CAD build for the part. Positions are in the model's coordinates, mm. A direction names the side the tool comes from. Round coordinates to 2 decimals unless told otherwise and drop trailing zeros. Loops run counter-clockwise (first coordinate to the right, second up) from the corner with the lowest first, then second, coordinate; pieces in that order, holes last.
```python
from build123d import *

# Parameters (mm, degrees)
SKETCH1_R             = 8.5
SKETCH1_R_2           = 6.5
BOSS_EXTRUDE1_DEPTH   = 9
SKETCH1_R_3           = 2.25
SKETCH1_R_4           = 0.75
BOSS_EXTRUDE1_2_DEPTH = 9
SKETCH2_R             = 9.5
BOSS_EXTRUDE2_DEPTH   = 1.5
SKETCH3_R             = 9.5
SKETCH3_R_2           = 6.5
BOSS_EXTRUDE3_DEPTH   = 1
BOSS_EXTRUDE4_REACH   = 19.051
CIRPATTERN1_COUNT     = 3
CUT_EXTRUDE2_START    = -2
SKETCH6_R             = 6.5
CUT_EXTRUDE2_DEPTH    = 2
FILLET1_R             = 3
BOSS_EXTRUDE5_START   = 1
SKETCH8_R             = 6.5
BOSS_EXTRUDE5_DEPTH   = 1
SKETCH11_R            = 8
BOSS_EXTRUDE6_DEPTH   = 2
SKETCH7_R             = 1
CUT_EXTRUDE3_DEPTH    = 7
FILLET2_R             = 1
CIRPATTERN2_COUNT     = 3
CUT_EXTRUDE4_START    = -20
SKETCH4_R             = 0.75
CUT_EXTRUDE4_DEPTH    = 20


with BuildPart() as part:
    # Sketch1 → Boss-Extrude1 (new body)
    with BuildSketch(Plane.XY):
        Circle(SKETCH1_R)
        Circle(SKETCH1_R_2, mode=Mode.SUBTRACT)
    extrude(amount=BOSS_EXTRUDE1_DEPTH)



with BuildPart() as body_2:
    # Sketch1 → Boss-Extrude1 2 (new body)
    with BuildSketch(Plane.XY):
        Circle(SKETCH1_R_3)
        Circle(SKETCH1_R_4, mode=Mode.SUBTRACT)
    extrude(amount=BOSS_EXTRUDE1_2_DEPTH)


with BuildPart() as part_1:
    add(part.part)

    add(body_2.part)  # Boss-Extrude2 merges body 2
    # Sketch2 → Boss-Extrude2 (add)
    with BuildSketch(Plane(origin=(0, 0, 0), x_dir=(-1, 0, 0), z_dir=(0, 0, -1))):
        Circle(SKETCH2_R)
    extrude(amount=BOSS_EXTRUDE2_DEPTH)

    # Sketch3 → Boss-Extrude3 (add)
    with BuildSketch(Plane.XY.offset(9)):
        Circle(SKETCH3_R)
        Circle(SKETCH3_R_2, mode=Mode.SUBTRACT)
    extrude(amount=BOSS_EXTRUDE3_DEPTH)

    # Sketch5 → Boss-Extrude4 (add, up to next)
    with BuildSketch(Plane.XY.offset(9), mode=Mode.PRIVATE) as boss_extrude4_sk1:
        with BuildLine():
            Line((2.25, 0), (6.5, 0))
            ThreePointArc((6.5, 0), (6.444391599, -0.848420249), (6.278517871, -1.682323793))
            Line((6.278517871, -1.682323793), (2.173333109, -0.582342851))
            ThreePointArc((2.173333109, -0.582342851), (2.230750938, -0.293683932), (2.25, 0))
        make_face()
    boss_extrude4_tool1 = extrude(boss_extrude4_sk1.sketch, amount=-BOSS_EXTRUDE4_REACH, mode=Mode.PRIVATE) - part_1.part
    boss_extrude4 = boss_extrude4_tool1.solids().sort_by_distance((4.665326, -0.614202, 9))[0]
    add(boss_extrude4)

    # CirPattern1: Boss-Extrude4 ×3 about axis
    cirpattern1_axis = Axis((0, 0, 0), (0, 0, 1))
    for i in range(1, CIRPATTERN1_COUNT):
        add(boss_extrude4.rotate(cirpattern1_axis, i * 360 / CIRPATTERN1_COUNT))

    # Sketch6 → Cut-Extrude2 (cut)
    with BuildSketch(Plane.XY.offset(9).offset(CUT_EXTRUDE2_START)):
        Circle(SKETCH6_R)
    extrude(amount=CUT_EXTRUDE2_DEPTH, mode=Mode.SUBTRACT)

    # Fillet1
    # the kernel refuses this fillet: 3 mm, written as the material it adds along each edge
    with BuildSketch(Plane(origin=(0, 0, 7), x_dir=(0.9659258262890711, -0.2588190451025104, 0), z_dir=(-0.2588190451025104, -0.9659258262890711, 0))) as fillet1_piece_1:
        with BuildLine():
            CenterArc((6.5 - FILLET1_R, FILLET1_R), FILLET1_R, 270, 90)
            Line((6.5 - FILLET1_R, 0), (6.5, 0))
            Line((6.5, 0), (6.5, FILLET1_R))
        make_face()
    revolve(axis=Axis((0, 0, 7), (0, 0, 1)), revolution_arc=15)
    with BuildSketch(Plane(origin=(0, 0, 7), x_dir=(-0.2588190451025142, 0.9659258262890701, 0), z_dir=(0.9659258262890701, 0.2588190451025142, 0))) as fillet1_piece_2:
        with BuildLine():
            CenterArc((6.5 - FILLET1_R, FILLET1_R), FILLET1_R, 270, 90)
            Line((6.5 - FILLET1_R, 0), (6.5, 0))
            Line((6.5, 0), (6.5, FILLET1_R))
        make_face()
    revolve(axis=Axis((0, 0, 7), (0, 0, 1)), revolution_arc=15)
    with BuildSketch(Plane(origin=(0, 0, 7), x_dir=(-0.7071067811865505, -0.7071067811865446, 0), z_dir=(-0.7071067811865446, 0.7071067811865505, 0))) as fillet1_piece_3:
        with BuildLine():
            CenterArc((6.5 - FILLET1_R, FILLET1_R), FILLET1_R, 270, 90)
            Line((6.5 - FILLET1_R, 0), (6.5, 0))
            Line((6.5, 0), (6.5, FILLET1_R))
        make_face()
    revolve(axis=Axis((0, 0, 7), (0, 0, 1)), revolution_arc=15)

    # Sketch8 → Boss-Extrude5 (add)
    with BuildSketch(Plane(origin=(0, 0, -1.5), x_dir=(-1, 0, 0), z_dir=(0, 0, -1)).offset(BOSS_EXTRUDE5_START)):
        Circle(SKETCH8_R)
    extrude(amount=-BOSS_EXTRUDE5_DEPTH)

    # Sketch11 → Boss-Extrude6 (add)
    with BuildSketch(Plane(origin=(0, 0, -2.5), x_dir=(-1, 0, 0), z_dir=(0, 0, -1))):
        Circle(SKETCH11_R)
    extrude(amount=BOSS_EXTRUDE6_DEPTH)

    # Sketch7 → Cut-Extrude3 (cut)
    with BuildSketch(Plane.XY):
        with Locations((1.722075446, -4.157457896)):
            Circle(SKETCH7_R)
    cut_extrude3 = extrude(amount=-CUT_EXTRUDE3_DEPTH, mode=Mode.SUBTRACT)

    # Fillet2
    # the kernel refuses this fillet: 1 mm, written as the material it adds along each edge
    with BuildSketch(Plane(origin=(0, 0, 0), x_dir=(0.9268638778365579, -0.37539759184333915, 0), z_dir=(-0.37539759184333915, -0.9268638778365579, 0))) as fillet2_piece_1:
        with BuildLine():
            CenterArc((6.5 - FILLET2_R, FILLET2_R), FILLET2_R, 270, 90)
            Line((6.5 - FILLET2_R, 0), (6.5, 0))
            Line((6.5, 0), (6.5, FILLET2_R))
        make_face()
    revolve(axis=Axis((0, 0, 0), (0, 0, 1)), revolution_arc=149.097777135)
    with BuildSketch(Plane(origin=(-0.25, 0, 0), x_dir=(0, 0, 1), z_dir=(1, 0, 0))) as fillet2_piece_2_section:
        with BuildLine():
            CenterArc((FILLET2_R, -FILLET2_R), FILLET2_R, 90, 90)
            Line((0, -FILLET2_R), (0, 0))
            Line((0, 0), (FILLET2_R, 0))
        make_face()
    fillet2_piece_2 = extrude(amount=9.25, mode=Mode.PRIVATE)
    fillet2_piece_2 = fillet2_piece_2 & Plane(origin=(0, 0, 0.222961637), x_dir=(1, 0, 0), z_dir=(0, 0, -1)) * Cylinder(6.5, 23, mode=Mode.PRIVATE)
    fillet2_piece_2 = fillet2_piece_2 - Plane(origin=(0, 0, 0.222961637), x_dir=(1, 0, 0), z_dir=(0, 0, -1)) * Cylinder(0.75, 23, mode=Mode.PRIVATE)
    add(fillet2_piece_2)
    with BuildSketch(Plane(origin=(8.693332437, -2.329371406, 0), x_dir=(-0.25881904510252135, -0.9659258262890682, 0), z_dir=(-0.9659258262890682, 0.25881904510252135, 0))) as fillet2_piece_3_section:
        with BuildLine():
            CenterArc((FILLET2_R, FILLET2_R), FILLET2_R, 180, 90)
            Line((0, FILLET2_R), (0, 0))
            Line((0, 0), (FILLET2_R, 0))
        make_face()
    fillet2_piece_3 = extrude(amount=9.25, mode=Mode.PRIVATE)
    fillet2_piece_3 = fillet2_piece_3 & Plane(origin=(0, 0, 0.22296165), x_dir=(1, 0, 0), z_dir=(0, 0, -1)) * Cylinder(8.5, 23, mode=Mode.PRIVATE)
    fillet2_piece_3 = fillet2_piece_3 - Plane(origin=(0, 0, 0.22296165), x_dir=(1, 0, 0), z_dir=(0, 0, -1)) * Cylinder(0.75, 23, mode=Mode.PRIVATE)
    add(fillet2_piece_3)
    with BuildSketch(Plane(origin=(0, 0, 0), x_dir=(-0.138328087862445, 0.9903864599782852, 0), z_dir=(0.9903864599782852, 0.138328087862445, 0))) as fillet2_piece_4:
        with BuildLine():
            CenterArc((6.5 - FILLET2_R, FILLET2_R), FILLET2_R, 270, 90)
            Line((6.5 - FILLET2_R, 0), (6.5, 0))
            Line((6.5, 0), (6.5, FILLET2_R))
        make_face()
    revolve(axis=Axis((0, 0, 0), (0, 0, 1)), revolution_arc=149.097777135)
    with BuildSketch(Plane(origin=(0, 0, 0), x_dir=(0.5547978045957125, 0.8319852138204006, 0), z_dir=(0.8319852138204006, -0.5547978045957125, 0))) as fillet2_piece_5:
        with BuildLine():
            CenterArc((2.25 + FILLET2_R, FILLET2_R), FILLET2_R, 180, 90)
            Line((2.25 + FILLET2_R, 0), (2.25, 0))
            Line((2.25, 0), (2.25, FILLET2_R))
        make_face()
    revolve(axis=Axis((0, 0, 0), (0, 0, 1)), revolution_arc=232.393578389)
    with BuildSketch(Plane(origin=(0.125, -0.216506351, 0), x_dir=(0, 0, 1), z_dir=(-0.49999999999999983, 0.8660254037844388, 0))) as fillet2_piece_6_section:
        with BuildLine():
            CenterArc((FILLET2_R, -FILLET2_R), FILLET2_R, 90, 90)
            Line((0, -FILLET2_R), (0, 0))
            Line((0, 0), (FILLET2_R, 0))
        make_face()
    fillet2_piece_6 = extrude(amount=9.25, mode=Mode.PRIVATE)
    fillet2_piece_6 = fillet2_piece_6 & Plane(origin=(0, 0, 0.222961635), x_dir=(1, 0, 0), z_dir=(0, 0, -1)) * Cylinder(6.5, 23, mode=Mode.PRIVATE)
    fillet2_piece_6 = fillet2_piece_6 - Plane(origin=(0, 0, 0.222961635), x_dir=(1, 0, 0), z_dir=(0, 0, -1)) * Cylinder(0.75, 23, mode=Mode.PRIVATE)
    add(fillet2_piece_6)
    with BuildSketch(Plane(origin=(-2.329371406, 8.693332437, 0), x_dir=(0, 0, 1), z_dir=(0.25881904510251996, -0.9659258262890685, 0))) as fillet2_piece_7_section:
        with BuildLine():
            CenterArc((FILLET2_R, -FILLET2_R), FILLET2_R, 90, 90)
            Line((0, -FILLET2_R), (0, 0))
            Line((0, 0), (FILLET2_R, 0))
        make_face()
    fillet2_piece_7 = extrude(amount=9.25, mode=Mode.PRIVATE)
    fillet2_piece_7 = fillet2_piece_7 & Plane(origin=(0, 0, 0.222961632), x_dir=(1, 0, 0), z_dir=(0, 0, -1)) * Cylinder(6.5, 23, mode=Mode.PRIVATE)
    fillet2_piece_7 = fillet2_piece_7 - Plane(origin=(0, 0, 0.222961632), x_dir=(1, 0, 0), z_dir=(0, 0, -1)) * Cylinder(0.75, 23, mode=Mode.PRIVATE)
    add(fillet2_piece_7)
    with BuildSketch(Plane(origin=(0, 0, 0), x_dir=(-0.7885357899741134, -0.614988868134945, 0), z_dir=(-0.614988868134945, 0.7885357899741134, 0))) as fillet2_piece_8:
        with BuildLine():
            CenterArc((6.5 - FILLET2_R, FILLET2_R), FILLET2_R, 270, 90)
            Line((6.5, FILLET2_R), (6.5, 0))
            Line((6.5, 0), (6.5 - FILLET2_R, 0))
        make_face()
    revolve(axis=Axis((0, 0, 0), (0, 0, 1)), revolution_arc=149.097777135)
    with BuildSketch(Plane(origin=(0, 0, 0), x_dir=(-0.9979192330393512, 0.06447638583352278, 0), z_dir=(0.06447638583352278, 0.9979192330393512, 0))) as fillet2_piece_9:
        with BuildLine():
            CenterArc((2.25 + FILLET2_R, FILLET2_R), FILLET2_R, 180, 90)
            Line((2.25, FILLET2_R), (2.25, 0))
            Line((2.25, 0), (2.25 + FILLET2_R, 0))
        make_face()
    revolve(axis=Axis((0, 0, 0), (0, 0, 1)), revolution_arc=232.393578389)
    with BuildSketch(Plane(origin=(0.125, 0.216506351, 0), x_dir=(0.8660254037844384, -0.5000000000000004, 0), z_dir=(-0.5000000000000004, -0.8660254037844384, 0))) as fillet2_piece_10_section:
        with BuildLine():
            CenterArc((FILLET2_R, FILLET2_R), FILLET2_R, 180, 90)
            Line((0, FILLET2_R), (0, 0))
            Line((0, 0), (FILLET2_R, 0))
        make_face()
    fillet2_piece_10 = extrude(amount=9.25, mode=Mode.PRIVATE)
    fillet2_piece_10 = fillet2_piece_10 & Plane(origin=(0, 0, 0.222961624), x_dir=(1, 0, 0), z_dir=(0, 0, -1)) * Cylinder(8.5, 23, mode=Mode.PRIVATE)
    fillet2_piece_10 = fillet2_piece_10 - Plane(origin=(0, 0, 0.222961624), x_dir=(1, 0, 0), z_dir=(0, 0, -1)) * Cylinder(0.75, 23, mode=Mode.PRIVATE)
    add(fillet2_piece_10)
    with BuildSketch(Plane(origin=(-6.363961031, -6.363961031, 0), x_dir=(0, 0, 1), z_dir=(0.7071067811865483, 0.7071067811865468, 0))) as fillet2_piece_11_section:
        with BuildLine():
            CenterArc((FILLET2_R, -FILLET2_R), FILLET2_R, 90, 90)
            Line((0, -FILLET2_R), (0, 0))
            Line((0, 0), (FILLET2_R, 0))
        make_face()
    fillet2_piece_11 = extrude(amount=9.25, mode=Mode.PRIVATE)
    fillet2_piece_11 = fillet2_piece_11 & Plane(origin=(0, 0, 0.22296162), x_dir=(1, 0, 0), z_dir=(0, 0, -1)) * Cylinder(6.5, 23, mode=Mode.PRIVATE)
    fillet2_piece_11 = fillet2_piece_11 - Plane(origin=(0, 0, 0.22296162), x_dir=(1, 0, 0), z_dir=(0, 0, -1)) * Cylinder(0.75, 23, mode=Mode.PRIVATE)
    add(fillet2_piece_11)
    with BuildSketch(Plane(origin=(0, 0, 0), x_dir=(0.44312142844363894, -0.8964615996539222, 0), z_dir=(-0.8964615996539222, -0.44312142844363894, 0))) as fillet2_piece_12:
        with BuildLine():
            CenterArc((2.25 + FILLET2_R, FILLET2_R), FILLET2_R, 180, 90)
            Line((2.25 + FILLET2_R, 0), (2.25, 0))
            Line((2.25, 0), (2.25, FILLET2_R))
        make_face()
    revolve(axis=Axis((0, 0, 0), (0, 0, 1)), revolution_arc=232.393578389)

    # CirPattern2: Cut-Extrude3 ×3 about axis
    cirpattern2_axis = Axis((0, 0, 0), (0, 0, 1))
    for i in range(1, CIRPATTERN2_COUNT):
        add(cut_extrude3.rotate(cirpattern2_axis, i * 360 / CIRPATTERN2_COUNT), mode=Mode.SUBTRACT)

    # Sketch4 → Cut-Extrude4 (cut)
    with BuildSketch(Plane.XY.offset(7).offset(CUT_EXTRUDE4_START)):
        with Locations(Location((0, 0, 0), (0, 0, 180))):
            Circle(SKETCH4_R)
    extrude(amount=CUT_EXTRUDE4_DEPTH, mode=Mode.SUBTRACT)

    # Sketch12 → Cut-Revolve1 (revolve, cut)
    with BuildSketch(Plane(origin=(0, 0, 0), x_dir=(1, 0, 0), z_dir=(0, 1, 0)), mode=Mode.PRIVATE) as cut_revolve1_sk:
        Polygon((6.5, 2.5), (10.5, 3.205307923), (10.5, 0.794692077), (6.5, 1.5), align=None)
    revolve(cut_revolve1_sk.sketch.rotate(Axis((0, 0, 0), (0, 0, -1)), 180), axis=Axis((0, 0, 0), (0, 0, -1)), mode=Mode.SUBTRACT)


solid = part_1.part
```
Item 1: Flat gauge pins, fed straight in: P1, Ø1.1, axis at x = 2, y = -4, coming from the +Z side; P2, Ø1.5, axis at x = 0, z = 2.5, coming from the -Y side; P3, Ø0.9, axis at x = -4.5, y = -1, coming from the +Z side; P4, Ø4, axis at y = 6.5, z = -1, coming from the +X side. Where does each tip first touch, or does it go through?
Answers follow:
P1: passes through
P2: stops at y = -8.5
P3: stops at z = 0
P4: stops at x = 8.37
Item 2: Cut at B-B, the plane z = 8.75. Give the cut face in (x, y) (3 decimals), plus the area to 3 significant figures.
Answers follow:
outline: circle Ø17 at (0, 0); hole (-4.596, -4.596) - (-4.403, -4.403) arc R6.227 ccw to (-3.114, -5.393) - (-3.25, -5.629) arc R6.5 ccw to (6.279, -1.682) - (6.015, -1.612) arc R6.227 ccw to (6.227, 0) - (6.5, 0) arc R6.5 ccw to (-1.682, 6.279) - (-1.612, 6.015) arc R6.227 ccw to (-3.114, 5.393) - (-3.25, 5.629) arc R6.5 ccw to start
area: 95.6 mm2
Item 3: Cut at A-A, the plane z = 3.5. Give the cut face in (x, y) (3 decimals).
Answers follow:
outline: circle Ø17 at (0, 0); hole (-4.596, -4.596) - (-1.591, -1.591) arc R2.25 cw to (-1.125, 1.949) - (-3.25, 5.629) arc R6.5 ccw to start; hole (-3.25, -5.629) arc R6.5 ccw to (6.279, -1.682) - (2.173, -0.582) arc R2.25 cw to (-1.125, -1.949) - close; hole (-1.682, 6.279) - (-0.582, 2.173) arc R2.25 cw to (2.25, 0) - (6.5, 0) arc R6.5 ccw to start; hole circle Ø1.5 at (0, 0)
Item 4: 3-axis set-ups, long thin cutter, end or side, ignore diameter. For faces 4 (the flat face through (0, -2, -4.5)), 5 (the flat face through (-2.2, -8.4, 9)), 6 (the cylindrical face through (0.83, -2.09, 3.96)): which of +Z, -Z, +X, -X, +Y, -Y reach the whole face in a straight line?
Answers follow:
face 4: -Z, +X, -X, +Y, -Y
face 5: none
face 6: +Z
Item 5: Two-plate mould, pull along Y, no slides. Class faces 1 (the cylindrical face through (2.41, -6.037, 5.437)), 2 (the flat face through (4, -6, 10)), 3 (the cylindrical face through (4.38, -8.43, 9.49)): released by +Y, released by -Y, zero draft, split by the parting line, or undercut.
Answers follow:
face 1: undercut
face 2: zero draft
face 3: split by the parting line
Item 6: Probe line 1 (X direction, y = 4.25, z = 0.75); line 2 (X direction, y = 4, z = 3); line 3 (Y direction, x = 3, z = 4.25). List the from-to ranges inside material, lowest first.
Answers follow:
line 1: x = -7.36 to -4.88, -2.49 to -1.11, 4.88 to 7.36
line 2: x = -7.5 to -5.12, -2.31 to -1.07, 5.12 to 7.5
line 3: y = -7.95 to -5.77, -0.8 to 0, 5.77 to 7.95
